Could you check a few things on this model? Use its own coordinates, in mm. A direction names the side the tool comes from. Round coordinates to 2 decimals unless told otherwise and drop trailing zeros. Loops run counter-clockwise (first coordinate to the right, second up) from the corner with the lowest first, then second, coordinate; pieces in that order, holes last. Notation, with made-up numbers: M 31,10.25 L 56,10.25 A31 ccw 56,34.25 Z; hole C 0,-32 d10. An arc over 180 degrees is marked long. Answer in a Markdown table with one row per item.
```python
from build123d import *

# Parameters (mm, degrees)
SKETCH1_R                = 1.5
SKETCH1_R_2              = 13
SKETCH1_R_3              = 2
BOSS_EXTRUDE1_DEPTH      = 6
SKETCH2_W                = 170
SKETCH2_H                = 3
BOSS_EXTRUDE2_DEPTH      = 15
BOSS_EXTRUDE2_DEPTH_BACK = 6
SKETCH3_R                = 2
CUT_EXTRUDE1_DEPTH       = 15


with BuildPart() as part:
    # Sketch1 → Boss-Extrude1 (new body)
    with BuildSketch(Plane.XY):
        Polygon((50, 5), (-50, 5), (-80, -15), (-120, -15), (-120, -55), (-43, -55), (0, -5), (43, -55), (50, -55), align=None)
        Polygon((43, -5), (43, -44.264450265), (9.232572773, -5), align=None, mode=Mode.SUBTRACT)
        with Locations((-107.875, -48.63990011)):
            Circle(SKETCH1_R, mode=Mode.SUBTRACT)
        with Locations((-92.125, -48.63990011)):
            Circle(SKETCH1_R, mode=Mode.SUBTRACT)
        with Locations((-115.75, -35)):
            Circle(SKETCH1_R, mode=Mode.SUBTRACT)
        with Locations((-100, -35)):
            Circle(SKETCH1_R_2, mode=Mode.SUBTRACT)
        with Locations((-84.25, -35)):
            Circle(SKETCH1_R, mode=Mode.SUBTRACT)
        Polygon((-80, -46.571581383), (-80, -25), (-50, -5), (-50, -46.571581383), align=None, mode=Mode.SUBTRACT)
        Polygon((-43, -44.264450265), (-43, -5), (-9.232572773, -5), align=None, mode=Mode.SUBTRACT)
        with Locations((-107.875, -21.36009989)):
            Circle(SKETCH1_R, mode=Mode.SUBTRACT)
        with Locations((-92.125, -21.36009989)):
            Circle(SKETCH1_R, mode=Mode.SUBTRACT)
        with Locations((-35, 0)):
            Circle(SKETCH1_R_3, mode=Mode.SUBTRACT)
        with Locations((35, 0)):
            Circle(SKETCH1_R_3, mode=Mode.SUBTRACT)
    extrude(amount=BOSS_EXTRUDE1_DEPTH)

    # Sketch2 → Boss-Extrude2 (add, two sides)
    with BuildSketch(Plane.XY.offset(6)) as boss_extrude2_sk:
        with Locations((-35, -56.5)):
            Rectangle(SKETCH2_W, SKETCH2_H)
    extrude(amount=BOSS_EXTRUDE2_DEPTH)
    extrude(boss_extrude2_sk.sketch, amount=-BOSS_EXTRUDE2_DEPTH_BACK)

    # Sketch3 → Cut-Extrude1 (cut)
    with BuildSketch(Plane(origin=(0, -55, 0), x_dir=(1, 0, 0), z_dir=(0, 1, 0))):
        with Locations((0, -13.5)):
            Circle(SKETCH3_R)
        with Locations((-50, -13.5)):
            Circle(SKETCH3_R)
        with Locations((-100, -13.5)):
            Circle(SKETCH3_R)
    extrude(amount=-CUT_EXTRUDE1_DEPTH, mode=Mode.SUBTRACT)


solid = part.part
```
1) I want a section at B-B, the plane y = -31. Please give me the cut outline in (x, z).
Computed:
| item | result |
|---|---|
| outline | M -120,0 L -112.37,0 L -112.37,6 L -120,6 Z; M -87.63,0 L -80,0 L -80,6 L -87.63,6 Z; M -50,0 L -43,0 L -43,6 L -50,6 Z; M -31.59,0 L -22.36,0 L -22.36,6 L -31.59,6 Z; M 22.36,0 L 31.59,0 L 31.59,6 L 22.36,6 Z; M 43,0 L 50,0 L 50,6 L 43,6 Z |
2) Which directions (+Z, -Z, +X, -X, +Y, -Y) give clear straight access to the entire face, cutting with the end or side of a thin tool? Please do faces 4 (the face through (-36, -58, 11)), 5 (the face through (-65, -15, 3)), 6 (the face through (-36, -55, 13)).
Computed:
| item | result |
|---|---|
| face 4 | +Z, -Z, +X, -X, -Y |
| face 5 | +Z, -Z |
| face 6 | +Z |
3) If we mould it in two halves opening along X, with no side actions, what happens to faces 1 (the face through (-120, -42, 4)), 2 (the face through (-100, -15, 3)), 3 (the face through (-117.25, -34.93, 2.96))? For each: released by +X, released by -X, zero draft, split by the parting line, or undercut.
Computed:
| item | result |
|---|---|
| face 1 | released by -X |
| face 2 | zero draft |
| face 3 | undercut |
4) I want a section at D-D, the plane y = -40. Please give me the cut outline in (x, z).
Computed:
| item | result |
|---|---|
| outline | M -120,0 L -112,0 L -112,6 L -120,6 Z; M -88,0 L -80,0 L -80,6 L -88,6 Z; M -50,0 L -43,0 L -43,6 L -50,6 Z; M -39.33,0 L -30.1,0 L -30.1,6 L -39.33,6 Z; M 30.1,0 L 39.33,0 L 39.33,6 L 30.1,6 Z; M 43,0 L 50,0 L 50,6 L 43,6 Z |
5) I want a section at A-A, the plane x = -84.25. Please give me the cut outline in (y, z).
Computed:
| item | result |
|---|---|
| outline | M -58,0 L -36.5,0 L -36.5,6 L -55,6 L -55,21 L -58,21 Z; M -33.5,0 L -15,0 L -15,6 L -33.5,6 Z |
6) I need wall thicknesses on line 1 (Y direction, x = -84.25, z = 2.55); line 2 (X direction, y = -16.5, z = 2.75); line 3 (X direction, y = -45, z = 5.25). Which ranges of each line are inside material? Lowest first, please.
Computed:
| item | result |
|---|---|
| line 1 | y = -58 to -36.5, -33.5 to -15 |
| line 2 | x = -120 to -67.25, -50 to -43, -19.12 to -9.89, 9.89 to 19.12, 43 to 50 |
| line 3 | x = -120 to -108.31, -91.69 to -80, -50 to -34.4, 34.4 to 50 |
7) I want a section at C-C, the plane x = 35. Please give me the cut outline in (y, z), plus the area to 3 significant figures.
Computed:
| item | result |
|---|---|
| outline | M -58,0 L -55,0 L -55,21 L -58,21 Z; M -45.7,0 L -34.96,0 L -34.96,6 L -45.7,6 Z; M -5,0 L -2,0 L -2,6 L -5,6 Z; M 2,0 L 5,0 L 5,6 L 2,6 Z |
| area | 163 mm² |
8) Will these pins go through, and if not, where does the flat tip stop? P1, Ø4, axis at x = -115.75, y = -35, coming from the +Z side; P2, Ø5, axis at x = -58, z = 3, coming from the +Y side; P3, Ø4, axis at x = -92.12, y = -21.36, coming from the -Z side; P4, Ø6.5, axis at x = -71, z = 13, coming from the +Y side.
Computed:
| item | result |
|---|---|
| P1 | stops at z = 6 |
| P2 | stops at y = 1.33 |
| P3 | stops at z = 0 |
| P4 | stops at y = -55 |
